from build123d import *

# Parameters (mm, degrees)
SKETCH1_W           = 90
SKETCH1_H           = 70
BOSS_EXTRUDE1_DEPTH = 40
SKETCH4_R           = 20
CUT_EXTRUDE1_DEPTH  = 40
SKETCH5_W           = 14.755351209
SKETCH5_H           = 65
CUT_EXTRUDE2_DEPTH  = 40
SKETCH6_W           = 12
SKETCH6_H           = 27.02325336
CUT_EXTRUDE3_DEPTH  = 40


with BuildPart() as part:
    # Sketch1 → Boss-Extrude1 (new body)
    with BuildSketch(Plane(origin=(0, 0, 0), x_dir=(1, 0, 0), z_dir=(0, 1, 0))):
        Rectangle(SKETCH1_W, SKETCH1_H)
    extrude(amount=BOSS_EXTRUDE1_DEPTH)

    # Sketch4 → Cut-Extrude1 (cut)
    with BuildSketch(Plane(origin=(0, 40, 0), x_dir=(1, 0, 0), z_dir=(0, 1, 0))):
        with Locations(Location((0, 5, 0), (0, 0, 270))):
            Circle(SKETCH4_R)
    extrude(amount=-CUT_EXTRUDE1_DEPTH, mode=Mode.SUBTRACT)

    # Sketch5 → Cut-Extrude2 (cut)
    with BuildSketch(Plane(origin=(0, 40, 0), x_dir=(1, 0, 0), z_dir=(0, 1, 0))):
        with Locations((-37.622324396, 2.5)):
            Rectangle(SKETCH5_W, SKETCH5_H)
        with Locations((37.622324396, 2.5)):
            Rectangle(SKETCH5_W, SKETCH5_H)
    extrude(amount=-CUT_EXTRUDE2_DEPTH, mode=Mode.SUBTRACT)

    # Sketch6 → Cut-Extrude3 (cut)
    with BuildSketch(Plane(origin=(0, 40, 0), x_dir=(1, 0, 0), z_dir=(0, 1, 0))):
        with Locations((0, 35)):
            Rectangle(SKETCH6_W, SKETCH6_H)
    extrude(amount=-CUT_EXTRUDE3_DEPTH, mode=Mode.SUBTRACT)


solid = part.part
CAD build for the part. Positions are in the model's coordinates, mm. A direction names the side the tool comes from. Round coordinates to 2 decimals unless told otherwise and drop trailing zeros. Loops run counter-clockwise (first coordinate to the right, second up) from the corner with the lowest first, then second, coordinate; pieces in that order, holes last. Notation, with made-up numbers: M -21.5,37.5 L 33.5,37.5 A28 cw 33.5,69.5 Z; hole C 20.25,-25.75 d6. An arc over 180 degrees is marked long. One line per question, with ' | ' between items. Start each with the question number.
Item 1: Which spindle directions (+Z, -Z, +X, -X, +Y, -Y) get a long thin tool onto all of the face, cutting with end or side? Do faces 4 (the flat face through (-30.245, 20, -2)), 5 (the flat face through (38, 20, 30)), 6 (the flat face through (6, 20, -29)). Say none if no direction does.
Item 2: Cut at A-A, the plane z = -5. Write the cut outline in (x, y).
Item 3: Two-plate mould, pull along X, no slides. Class faces 1 (the flat face through (-45, 20, 33)), 2 (the flat face through (-38, 20, 30)), 3 (the cylindrical face through (-0.794, 20.28, 14.984)): pulls with the +X half, pulls with the -X half, needs draft (parallel to the pull), parting line crosses it, or undercut.
Item 4: Cut at B-B, the plane y = 9. Write the cut outline in (x, z).
Item 5: Pin check, flat tips, straight feed: pin 1 Ø5.5 at (y, z) = (10.5, -31.5) entering from +X; pin 2 Ø6 at (x, z) = (-20.5, -5.5) entering from -Y; pin 3 Ø4.5 at (x, y) = (-40.5, 23.5) entering from -Z; pin 4 Ø1.5 at (y, z) = (22.5, -18) entering from -X. Stop position of each tip, or through.
Item 6: Cut at D-D, the plane z = 20. Write the cut outline in (x, y), plus the area to 3 significant figures.
Item 7: Cut at C-C, the plane x = -13. Write the cut outline in (y, z).
Item 8: Wall check: line 1 (X direction, y = 16, z = -5); line 2 (X direction, y = 22.5, z = -26.5); line 3 (X direction, y = 4, z = 25.5). Give the ranges that are in metal, low to high.
Responses:
1) face 4: -Z, -X, +Y, -Y | face 5: -Z, +X, +Y, -Y | face 6: -Z, +Y, -Y
2) outline: M -30.24,0 L -20,0 L -20,40 L -30.24,40 Z; M 20,0 L 30.24,0 L 30.24,40 L 20,40 Z
3) face 1: pulls with the -X half | face 2: needs draft | face 3: undercut
4) outline: M -45,30 L -30.24,30 L -30.24,-35 L -6,-35 L -6,-24.08 A20 cw long 6,-24.08 L 6,-35 L 30.24,-35 L 30.24,30 L 45,30 L 45,35 L -45,35 Z
5) pin 1: stops at x = 30.24 | pin 2: stops at y = 0 | pin 3: stops at z = 30 | pin 4: stops at x = -30.24
6) outline: M -30.24,0 L 30.24,0 L 30.24,40 L -30.24,40 Z | area: 2,420 mm²
7) outline: M 0,-35 L 40,-35 L 40,-20.2 L 0,-20.2 Z; M 0,10.2 L 40,10.2 L 40,35 L 0,35 Z
8) line 1: x = -30.24 to -20, 20 to 30.24 | line 2: x = -30.24 to -6, 6 to 30.24 | line 3: x = -30.24 to 30.24
